Source: CAD feature listing. Evaluate the final solid. Frame: model axes, mm. Face numbers are marked on the shaded views. Give positions to 0.01 mm unless a question says otherwise; leave off trailing zeros. Write each loop counter-clockwise with the first axis right and the second up, starting at its lowest first coordinate (ties: lowest second). Pieces come first, ordered by that corner, then holes.
```python
from build123d import *

# Parameters (mm, degrees)
F1_DEPTH = 1308


with BuildPart() as f1:
    # F0 (on Front) → F1 (new body)
    with BuildSketch(Plane.XZ):
        with BuildLine():
            Line((-25.16784, 62.5), (-25.16784, -62.5))
            Line((-25.16784, -62.5), (39.83216, -62.5))
            Line((39.83216, -62.5), (39.83216, -55))
            Line((39.83216, -55), (-12.46784, -55))
            ThreePointArc((-12.46784, -55), (-18.124695, -52.656854), (-20.46784, -47))
            Line((-20.46784, -47), (-20.46784, 47))
            ThreePointArc((-20.46784, 47), (-18.124695, 52.656854), (-12.46784, 55))
            Line((-12.46784, 55), (39.83216, 55))
            Line((39.83216, 55), (39.83216, 62.5))
            Line((39.83216, 62.5), (-25.16784, 62.5))
        make_face()
    extrude(amount=F1_DEPTH)


solid = f1.part
```
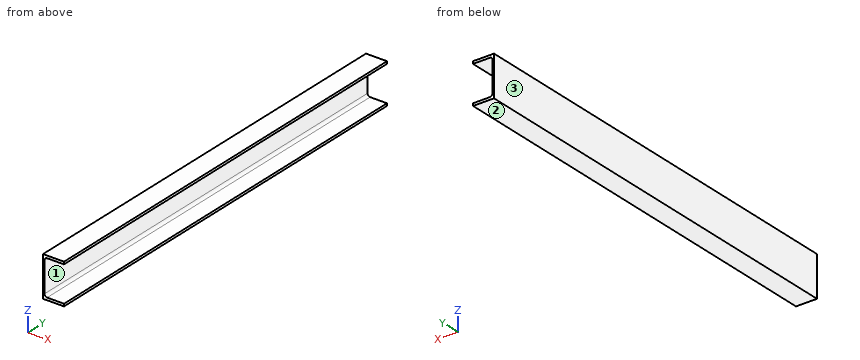
1. Pin query (flat end, axial travel): P1, Ø12, axis at x = -6, z = 46, coming from the +Y side; P2, Ø1, axis at y = -982.5, z = 32, coming from the +X side. Return the tip coordinate at first contact, or that it passes through.
2. Line query: probe 1 along Z at (x, y) = (26.5, -579); probe 2 along Z at (x, y) = (-14, -1200); probe 3 along X at (y, z) = (-192, -20). Output: solid intervals per line, ascending.
3. Section query A-A (x = 19.5). Return loops of the section in (y, z), plus the area to 3 significant figures.
4. Pull-direction query (X, two-part tool) for the marked faces 1, 2 and 3; classes: pulls with the +X half, pulls with the -X half, needs draft (parallel to the pull), parting line crosses it, or undercut.
5. Section query B-B (y = -151). Return loops of the section in (x, z), plus the area to 3 significant figures.
6. Section query C-C (z = -4.5). Return loops of the section in (x, y), plus the area to 3 significant figures.
The answers:
1. P1: passes through
1. P2: stops at x = -20.47
2. probe 1: z = -62.5 to -55, 55 to 62.5
2. probe 2: z = -62.5 to -54.85, 54.85 to 62.5
2. probe 3: x = -25.17 to -20.47
3. outline: (-1308, -62.5) - (0, -62.5) - (0, -55) - (-1308, -55) - close; (-1308, 55) - (0, 55) - (0, 62.5) - (-1308, 62.5) - close
3. area: 19,600 mm2
4. face 1: pulls with the +X half
4. face 2: needs draft
4. face 3: pulls with the -X half
5. outline: (-25.17, -62.5) - (39.83, -62.5) - (39.83, -55) - (-12.47, -55) arc R8 cw to (-20.47, -47) - (-20.47, 47) arc R8 cw to (-12.47, 55) - (39.83, 55) - (39.83, 62.5) - (-25.17, 62.5) - close
5. area: 1,520 mm2
6. outline: (-25.17, -1308) - (-20.47, -1308) - (-20.47, 0) - (-25.17, 0) - close
6. area: 6,150 mm2
